Can you work these out from the model? Positions are in its coordinate system, mm. A direction names the side the tool comes from. Round coordinates to 2 decimals unless told otherwise and drop trailing zeros. Loops run counter-clockwise (first coordinate to the right, second up) from the corner with the lowest first, then second, coordinate; pieces in that order, holes last. Notation, with made-up numbers: M 84,64.25 L 103,64.25 A12 cw 103,83.25 Z; hole C 30.5,69 d9. An arc over 180 degrees is marked long. Return JSON: item names as keys, results as strings.
```python
from build123d import *

# Parameters (mm, degrees)
F0_W     = 40
F0_H     = 10
F1_DEPTH = 10
F3_DEPTH = 40
F4_W     = 15
F4_H     = 10.352762
F5_DEPTH = 1
F6_W     = 40
F6_H     = 0.72
F7_DEPTH = 9
F8_R     = 1
F9_SIZE  = 2


with BuildPart() as f1:
    # F0 (on Top) → F1 (new body)
    with BuildSketch(Plane.XY):
        Rectangle(F0_W, F0_H)
    extrude(amount=F1_DEPTH)

    # F2 (on face) → F3 (join, through all)
    with BuildSketch(Plane.YZ.offset(20)):
        Polygon((-5, 10), (5, 10), (-5, 12.679492), align=None)
    extrude(amount=-F3_DEPTH)

    # F4 (on face) → F5 (join)
    with BuildSketch(Plane(origin=(0, 2.834936, 10.580127), x_dir=(1, 0, 0), z_dir=(0, 0.258819, 0.965926))):
        with Locations((0, -2.934942)):
            Rectangle(F4_W, F4_H)
    extrude(amount=F5_DEPTH)

    # F6 (on face) → F7 (cut)
    with BuildSketch(Plane(origin=(0, 0, 0), x_dir=(1, 0, 0), z_dir=(0, 0, -1))):
        Rectangle(F6_W, F6_H)
    extrude(amount=-F7_DEPTH, mode=Mode.SUBTRACT)

    # F8
    f8_edges = [f1.edges().sort_by_distance(p)[0] for p in [
        (0, -0.36, 0),
        (0, 0.36, 0),
    ]]
    fillet(f8_edges, radius=F8_R)

    # F9
    f9_edges = [f1.edges().sort_by_distance(p)[0] for p in [
        (20, 5, 5),
        (-20, 5, 5),
    ]]
    chamfer(f9_edges, length=F9_SIZE)


solid = f1.part
```
Q1. Thinking about a two-plate mould opening in Z: for faces 6 (the flat face through (0, -5, 6)), 7 (the flat face through (-0.1, -4.87, 13.16)), 8 (the flat face through (0, -3, 0)), which applies, pulls with the +Z half, pulls with the -Z half, needs draft (parallel to the pull), parting line crosses it, or undercut?
Results:
{"face 6": "needs draft", "face 7": "pulls with the +Z half", "face 8": "pulls with the -Z half"}
Q2. I'm going to push flat-ended pins straight in: pin 1 Ø1.1 at (y, z) = (-1.5, 12.5) entering from +X; pin 2 Ø8 at (x, z) = (2.5, 3.5) entering from +Y; pin 3 Ø0.6 at (x, y) = (-2.5, 0) entering from -Z. Where does each tip first touch, or does it pass through?
Results:
{"pin 1": "stops at x = 7.5", "pin 2": "stops at y = 5", "pin 3": "stops at z = 9"}
Q3. If I drill on line 1 along Y through (x, z) = (-11, 7); line 2 along Y through (x, z) = (1, 9.5); line 3 along Z through (x, y) = (-2, 2), over which ranges is the centre line in solid material (lowest first)?
Results:
{"line 1": "y = -5 to -0.36, 0.36 to 5", "line 2": "y = -5 to 5", "line 3": "z = 0 to 11.84"}
Q4. Suppose I cut it at D-D, the plane x = 11. Please give me the cut outline in (y, z).
Results:
{"outline": "M -5,0 L -1.36,0 A1 ccw -0.36,1 L -0.36,9 L 0.36,9 L 0.36,1 A1 ccw 1.36,0 L 5,0 L 5,10 L -5,12.68 Z"}
Q5. Suppose I cut it at C-C, the plane y = -3.75. Please give me the cut outline in (x, z), plus the area to 3 significant figures.
Results:
{"outline": "M -20,0 L 20,0 L 20,12.34 L 7.5,12.34 L 7.5,13.38 L -7.5,13.38 L -7.5,12.34 L -20,12.34 Z", "area": "509 mm2"}
Q6. Suppose I cut it at A-A, the plane z = 8. Please give me the cut outline in (x, y), plus the area to 3 significant figures.
Results:
{"outline": "M -20,-5 L 20,-5 L 20,-0.36 L -20,-0.36 Z; M -20,0.36 L 20,0.36 L 20,3 L 18,5 L -18,5 L -20,3 Z", "area": "367 mm2"}
Q7. On a 3-axis mill with a long thin cutter (end or side, diameter ignored), from which of +Z, -Z, +X, -X, +Y, -Y can I reach the whole of each face in a straight line? I mean faces 1 (the flat face through (0, 0.36, 5)), 2 (the flat face through (-7.5, 0, 12)), 3 (the flat face through (0, 3, 0)), 4 (the flat face through (0, 5, 5)), 5 (the flat face through (7.5, 0, 12)). Say none if no direction works.
Results:
{"face 1": "-Z, +X, -X", "face 2": "+Z, -X, +Y", "face 3": "-Z, +X, -X, +Y, -Y", "face 4": "-Z, +X, -X, +Y", "face 5": "+Z, +X, +Y"}
